Work out the finished part from the listing and answer in its coordinate system (mm). Face numbers are marked on the shaded views. Round coordinates to 2 decimals unless told otherwise and drop trailing zeros. Loops run counter-clockwise (first coordinate to the right, second up) from the corner with the lowest first, then second, coordinate; pieces in that order, holes last.
```python
from build123d import *

# Parameters (mm, degrees)
CROQUIS1_R              = 63
CROQUIS1_R_2            = 44.5
CROQUIS1_R_3            = 2.25
SALIENTE_EXTRUIR1_DEPTH = 8
CROQUIS2_R              = 48
CORTAR_EXTRUIR1_DEPTH   = 3


with BuildPart() as part:
    # Croquis1 → Saliente-Extruir1 (new body)
    with BuildSketch(Plane(origin=(0, 0, 0), x_dir=(1, 0, 0), z_dir=(0, 1, 0))):
        with Locations(Location((0, 0, 0), (0, 0, 270))):
            Circle(CROQUIS1_R)
        with Locations(Location((0, 0, 0), (0, 0, 270))):
            Circle(CROQUIS1_R_2, mode=Mode.SUBTRACT)
        with Locations(Location((0, 55.5, 0), (0, 0, 270))):
            Circle(CROQUIS1_R_3, mode=Mode.SUBTRACT)
        with Locations(Location((48.06440991, 27.75, 0), (0, 0, 270))):
            Circle(CROQUIS1_R_3, mode=Mode.SUBTRACT)
        with Locations(Location((48.06440991, -27.75, 0), (0, 0, 270))):
            Circle(CROQUIS1_R_3, mode=Mode.SUBTRACT)
        with Locations(Location((0, -55.5, 0), (0, 0, 270))):
            Circle(CROQUIS1_R_3, mode=Mode.SUBTRACT)
        with Locations(Location((-48.06440991, -27.75, 0), (0, 0, 270))):
            Circle(CROQUIS1_R_3, mode=Mode.SUBTRACT)
        with Locations(Location((-48.06440991, 27.75, 0), (0, 0, 270))):
            Circle(CROQUIS1_R_3, mode=Mode.SUBTRACT)
    extrude(amount=SALIENTE_EXTRUIR1_DEPTH)

    # Croquis2 → Cortar-Extruir1 (cut)
    with BuildSketch(Plane.XZ):
        with Locations(Location((0, 0, 0), (0, 0, 270))):
            Circle(CROQUIS2_R)
    extrude(amount=-CORTAR_EXTRUIR1_DEPTH, mode=Mode.SUBTRACT)


solid = part.part
```
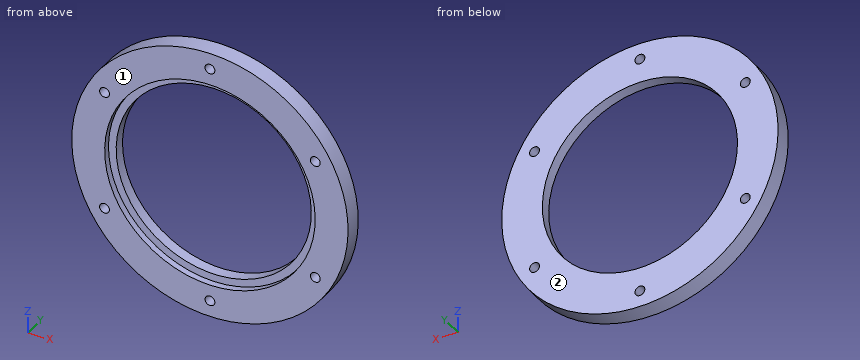
1. Consider probe 1 along X at (y, z) = (5.4, 0); probe 2 along X at (y, z) = (6.25, 27.75); probe 3 along X at (y, z) = (3.5, -27.5). Determine where each line is inside the solid, lowest interval first.
Answer key:
probe 1: x = -63 to -44.5, 44.5 to 63
probe 2: x = -56.56 to -50.31, -45.81 to -34.79, 34.79 to 45.81, 50.31 to 56.56
probe 3: x = -56.68 to -50.3, -45.83 to -34.99, 34.99 to 45.83, 50.3 to 56.68
2. Find section B-B (z = 17). Write down the section's boundary in (x, y), then the cut area to 3 significant figures.
Answer key:
outline: (-60.66, 0) - (-44.89, 0) - (-44.89, 3) - (-41.12, 3) - (-41.12, 8) - (-60.66, 8) - close; (41.12, 3) - (44.89, 3) - (44.89, 0) - (60.66, 0) - (60.66, 8) - (41.12, 8) - close
area: 290 mm2
3. Determine the mould class of the marked faces 1 and 2 for opening direction Y: +Y half, -Y half, draft (parallel to the pull), parting line (faces both ways), or undercut.
Answer key:
face 1: -Y half
face 2: +Y half
4. Find section D-D (z = -55.5). Write down the section's boundary in (x, y), then the cut area to 3 significant figures.
Answer key:
outline: (-29.81, 0) - (-2.25, 0) - (-2.25, 8) - (-29.81, 8) - close; (2.25, 0) - (29.81, 0) - (29.81, 8) - (2.25, 8) - close
area: 441 mm2
5. Given pin 1 (2 mm diameter, centred on x = -34, y = 6, fed in from +Z); pin 2 (4 mm diameter, centred on x = 1.5, y = 4, fed in from +Z); pin 3 (3 mm diameter, centred on y = 2, z = -20.5, fed in from +X); pin 4 (1.5 mm diameter, centred on y = 3, z = 29.5, fed in from +X), each flat-ended and moving along its own axis, determine where each tip first touches the part or whether it passes through.
Answer key:
pin 1: stops at z = 53.67
pin 2: stops at z = 63
pin 3: stops at x = 60.07
pin 4: stops at x = 56.06
6. Find section A-A (x = -10). Write down the section's boundary in (y, z).
Answer key:
outline: (0, -62.2) - (8, -62.2) - (8, -43.36) - (3, -43.36) - (3, -46.95) - (0, -46.95) - close; (0, 46.95) - (3, 46.95) - (3, 43.36) - (8, 43.36) - (8, 62.2) - (0, 62.2) - close
7. Find section C-C (y = 4.75). Write down the section's boundary in (x, z), then the cut area to 3 significant figures.
Answer key:
outline: circle Ø126 at (0, 0); hole circle Ø4.5 at (-48.06, -27.75); hole circle Ø4.5 at (-48.06, 27.75); hole circle Ø89 at (0, 0); hole circle Ø4.5 at (0, -55.5); hole circle Ø4.5 at (0, 55.5); hole circle Ø4.5 at (48.06, -27.75); hole circle Ø4.5 at (48.06, 27.75)
area: 6,150 mm2
